```python
from build123d import *

# Parameters (mm, degrees)
SKETCH_1_R          = 1.6
SKETCH_1_R_2        = 2.6
EXTRUDE_1_DEPTH     = 1.5
SKETCH_2_R          = 2.6
CUT_EXTRUDE_1_DEPTH = 253.257804636
SKETCH_3_W          = 35
SKETCH_3_H          = 30
CUT_EXTRUDE_2_DEPTH = 253.257804636
FILLET_1_R          = 5


with BuildPart() as part:
    # 草图1 → 凸台-拉伸1 (new, symmetric)
    with BuildSketch(Plane.XY):
        Polygon((-60, 20), (-60, -20), (60, -20), (60, 20), (10, 70), (10, 245), (-10, 245), (-10, 70), align=None)
        with Locations((-52.5, -14.5)):
            Circle(SKETCH_1_R, mode=Mode.SUBTRACT)
        with Locations((52.5, -14.5)):
            Circle(SKETCH_1_R, mode=Mode.SUBTRACT)
        with Locations((52.5, 14.5)):
            Circle(SKETCH_1_R, mode=Mode.SUBTRACT)
        with Locations((-52.5, 14.5)):
            Circle(SKETCH_1_R, mode=Mode.SUBTRACT)
        with Locations((0, 7.5)):
            Circle(SKETCH_1_R_2, mode=Mode.SUBTRACT)
        with Locations((0, -7.5)):
            Circle(SKETCH_1_R_2, mode=Mode.SUBTRACT)
    extrude(amount=EXTRUDE_1_DEPTH, both=True)

    # 草图2 → 切除-拉伸1 (cut, through all)
    with BuildSketch(Plane.XY.offset(1.5)):
        with Locations((0, 217.5)):
            Circle(SKETCH_2_R)
        with Locations((0, 187.5)):
            Circle(SKETCH_2_R)
        with Locations((0, 167.5)):
            Circle(SKETCH_2_R)
        with Locations((0, 122.5)):
            Circle(SKETCH_2_R)
        with Locations((0, 112.5)):
            Circle(SKETCH_2_R)
        with Locations((0, 102.5)):
            Circle(SKETCH_2_R)
        with Locations((0, 57.5)):
            Circle(SKETCH_2_R)
        with Locations((0, 37.5)):
            Circle(SKETCH_2_R)
    extrude(amount=-CUT_EXTRUDE_1_DEPTH, mode=Mode.SUBTRACT)

    # 草图3 → 切除-拉伸2 (cut, through all)
    with BuildSketch(Plane.XY.offset(1.5)):
        Polygon((-42, 29.514718626), (-12, 29.514718626), (-12, 59.514718626), align=None)
        with Locations((-29.5, 0)):
            Rectangle(SKETCH_3_W, SKETCH_3_H)
    cut_extrude_2 = extrude(amount=-CUT_EXTRUDE_2_DEPTH, mode=Mode.SUBTRACT)

    # 镜向1: 切除-拉伸2 across plane
    add(cut_extrude_2.mirror(Plane(origin=(0, 0, 0), x_dir=(0, 0, 1), z_dir=(1, 0, 0))), mode=Mode.SUBTRACT)

    # 圆角1
    fillet_1_edges = [part.edges().sort_by_distance(p)[0] for p in [
        (12, 59.514718626, 0),
        (42, 29.514718626, 0),
        (12, 29.514718626, 0),
        (12, 15, 0),
        (47, 15, 0),
        (47, -15, 0),
        (12, -15, 0),
        (60, -20, 0),
        (-60, -20, 0),
        (-60, 20, 0),
        (-10, 70, 0),
        (-10, 245, 0),
        (10, 245, 0),
        (10, 70, 0),
        (60, 20, 0),
        (-42, 29.514718626, 0),
        (-12, 59.514718626, 0),
        (-12, 29.514718626, 0),
        (-47, 15, 0),
        (-12, 15, 0),
        (-12, -15, 0),
        (-47, -15, 0),
    ]]
    fillet(fillet_1_edges, radius=FILLET_1_R)

    # 草图5 → M5 六角凹锥坑螺钉的锥形沉头孔1 (revolve, cut)
    with BuildSketch(Plane(origin=(0, -7.5, 1.5), x_dir=(0, -1, 0), z_dir=(1, 0, 0))):
        Polygon((0, 0), (0, 3), (2.75, 3), (2.75, 2.85), (5.6, 0), align=None)
    revolve(axis=Axis((0, -7.5, 7.85), (0, 0, -1)), mode=Mode.SUBTRACT)


solid = part.part
```
Input: part model. Units: mm. Frame: model coordinates. A direction names the side the tool comes from. Give positions to 0.01 mm unless a question says otherwise; leave off trailing zeros. Order: outer loops, then holes, each group sorted by start corner. A loop starts at its lowest first (then second) coordinate and runs counter-clockwise, first axis right, second up. Notation, with made-up numbers: (23, 57.5) - (58, 57.5) arc R6 cw to (58, 66.5) - close; hole circle Ø2 at (38, -11.75). An arc over 180 degrees is marked (long way). Put each result on its own line as item: value.
Item 1: Access query for faces 1 (the flat face through (26.909, 44.605, 0.021)), 2 (the cylindrical face through (-9, 243, 0)). Directions: +Z, -Z, +X, -X, +Y, -Y. A direction counts if a zero-diameter tool reaches every point of the face in a straight line with its end or side. Return the directions, or none.
Found:
face 1: +Z, -Z
face 2: +Z, -Z, -X, +Y
Item 2: Draft query along X for faces 3 (the cylindrical face through (46, 13, 0)), 4 (the flat face through (0, 84, -1.5)), 5 (the cylindrical face through (58, -19, 0)). Return one class per face: +X half, -X half, draft (parallel to the pull), parting line (faces both ways), or undercut.
Found:
face 3: undercut
face 4: draft
face 5: +X half
Item 3: Contact query for flat-ended pins moving along their axis: pin 1 (1.5 mm diameter, centred on x = -28, z = 0.5, fed in from +Y); pin 2 (1.5 mm diameter, centred on y = 80, z = -0.5, fed in from -X). Output: stop coordinate, or through.
Found:
pin 1: stops at y = 52.75
pin 2: stops at x = -10
Item 4: Section query A-A, the plane y = 122.5. Return loops of the section in (x, z), then the cut area to 3 significant figures.
Found:
outline: (-10, -1.5) - (-2.6, -1.5) - (-2.6, 1.5) - (-10, 1.5) - close; (2.6, -1.5) - (10, -1.5) - (10, 1.5) - (2.6, 1.5) - close
area: 44.4 mm^2
Item 5: Ray query, L1, parallel to X at y = -7.5, z = -1.4; L2, parallel to X at y = 10.5, z = -0.7; L3, parallel to X at y = 167.5, z = 0.2. Return the intervals inside material, ascending. Write a range as from..to.
Found:
L1: x = -60..-47, -12..-2.75, 2.75..12, 47..60
L2: x = -60..-46.97, -12.03..12.03, 46.97..60
L3: x = -10..-2.6, 2.6..10
Item 6: Section query C-C, the plane z = 1. Count the separate pieces of the cut face and the enclosed holes in it, then the cut area to 3 significant figures.
Found:
separate pieces: 1
enclosed holes: 18
area: 8,650 mm^2
Item 7: Section query B-B, the plane y = 7.5. Return loops of the section in (x, z).
Found:
outline: (-60, -1.5) - (-47, -1.5) - (-47, 1.5) - (-60, 1.5) - close; (-12, -1.5) - (-2.6, -1.5) - (-2.6, 1.5) - (-12, 1.5) - close; (2.6, -1.5) - (12, -1.5) - (12, 1.5) - (2.6, 1.5) - close; (47, -1.5) - (60, -1.5) - (60, 1.5) - (47, 1.5) - close
